```python
from build123d import *

# Parameters (mm, degrees)
BOSS_EXTRUDE1_DEPTH = 6
BOSS_EXTRUDE2_DEPTH = 1
BOSS_EXTRUDE3_START = 6
BOSS_EXTRUDE3_DEPTH = 6
SKETCH4_R           = 4
CUT_EXTRUDE1_DEPTH  = 0.7
SKETCH5_R           = 2
BOSS_EXTRUDE4_DEPTH = 0.7


with BuildPart() as part:
    # Sketch1 → Boss-Extrude1 (new body)
    with BuildSketch(Plane(origin=(0, 0, 0), x_dir=(1, 0, 0), z_dir=(0, 1, 0))):
        with BuildLine():
            ThreePointArc((-2.5, 7.282856582), (-7.7, 0), (-2.5, -7.282856582))
            Line((-2.5, -7.282856582), (-2.5, -6.216108107))
            ThreePointArc((-2.5, -6.216108107), (-6.7, 0), (-2.5, 6.216108107))
            Line((-2.5, 6.216108107), (-2.5, 7.282856582))
        make_face()
        with BuildLine():
            Line((-2.5, -6.216108107), (-2.5, -7.282856582))
            ThreePointArc((-2.5, -7.282856582), (0, -7.7), (2.5, -7.282856582))
            Line((2.5, -7.282856582), (2.5, -6.216108107))
            ThreePointArc((2.5, -6.216108107), (0, -6.7), (-2.5, -6.216108107))
        make_face()
        with BuildLine():
            Line((2.5, -6.216108107), (2.5, -7.282856582))
            ThreePointArc((2.5, -7.282856582), (6.266578014, -4.474371464), (7.7, 0))
            ThreePointArc((7.7, 0), (6.266578014, 4.474371464), (2.5, 7.282856582))
            Line((2.5, 7.282856582), (2.5, 6.216108107))
            ThreePointArc((2.5, 6.216108107), (5.551576353, 3.750999867), (6.7, 0))
            ThreePointArc((6.7, 0), (5.551576353, -3.750999867), (2.5, -6.216108107))
        make_face()
    extrude(amount=BOSS_EXTRUDE1_DEPTH)

    # Sketch2 → Boss-Extrude2 (add)
    with BuildSketch(Plane(origin=(0, 6, 0), x_dir=(1, 0, 0), z_dir=(0, 1, 0))):
        with BuildLine():
            Line((3, 13.7), (-3, 13.7))
            Line((-3, 13.7), (-7.191011254, 2.753063229))
            ThreePointArc((-7.191011254, 2.753063229), (-5.348708418, 5.539071968), (-2.5, 7.282856582))
            ThreePointArc((-2.5, 7.282856582), (0, 7.7), (2.5, 7.282856582))
            ThreePointArc((2.5, 7.282856582), (5.348708418, 5.539071968), (7.191011254, 2.753063229))
            Line((7.191011254, 2.753063229), (3, 13.7))
        make_face()
        with BuildLine():
            ThreePointArc((2.5, 6.216108107), (0, -6.7), (-2.5, 6.216108107))
            Line((-2.5, 6.216108107), (-2.5, 7.282856582))
            ThreePointArc((-2.5, 7.282856582), (0, -7.7), (2.5, 7.282856582))
            Line((2.5, 7.282856582), (2.5, 6.216108107))
        make_face()
        with BuildLine():
            ThreePointArc((-2.5, 7.282856582), (-5.348708418, 5.539071968), (-7.191011254, 2.753063229))
            ThreePointArc((-7.191011254, 2.753063229), (-1.399859519, -7.571683652), (7.7, 0))
            ThreePointArc((7.7, 0), (7.571683652, 1.399859519), (7.191011254, 2.753063229))
            ThreePointArc((7.191011254, 2.753063229), (5.348708418, 5.539071968), (2.5, 7.282856582))
            Line((2.5, 7.282856582), (2.5, 6.216108107))
            ThreePointArc((2.5, 6.216108107), (0, -6.7), (-2.5, 6.216108107))
            Line((-2.5, 6.216108107), (-2.5, 7.282856582))
        make_face()
        with BuildLine():
            ThreePointArc((2.5, 7.282856582), (0, 7.7), (-2.5, 7.282856582))
            Line((-2.5, 7.282856582), (-2.5, 6.216108107))
            ThreePointArc((-2.5, 6.216108107), (0, -6.7), (2.5, 6.216108107))
            Line((2.5, 6.216108107), (2.5, 7.282856582))
        make_face()
    extrude(amount=BOSS_EXTRUDE2_DEPTH)

    # Sketch3 → Boss-Extrude3 (add)
    with BuildSketch(Plane.XZ.offset(-6).offset(BOSS_EXTRUDE3_START)):
        with BuildLine():
            Line((-7.191011254, -2.753063229), (-3, -13.7))
            Line((-3, -13.7), (-1.929218753, -13.7))
            Line((-1.929218753, -13.7), (-2.5, -7.282856582))
            ThreePointArc((-2.5, -7.282856582), (-5.348708418, -5.539071968), (-7.191011254, -2.753063229))
        make_face()
        with BuildLine():
            Line((2.5, -7.282856582), (1.929218753, -13.7))
            Line((1.929218753, -13.7), (3, -13.7))
            Line((3, -13.7), (7.191011254, -2.753063229))
            ThreePointArc((7.191011254, -2.753063229), (5.348708418, -5.539071968), (2.5, -7.282856582))
        make_face()
    extrude(amount=-BOSS_EXTRUDE3_DEPTH)

    # Sketch4 → Cut-Extrude1 (cut)
    with BuildSketch(Plane(origin=(0, 7, 0), x_dir=(1, 0, 0), z_dir=(0, 1, 0))):
        Circle(SKETCH4_R)
        with BuildLine():
            Line((-2.031506006, 3.445719569), (-3.200269116, 4.473061322))
            ThreePointArc((-3.200269116, 4.473061322), (-3.889087297, 3.889087297), (-4.473061322, 3.200269116))
            Line((-4.473061322, 3.200269116), (-3.445719569, 2.031506006))
            ThreePointArc((-3.445719569, 2.031506006), (-2.828427125, 2.828427125), (-2.031506006, 3.445719569))
        make_face()
        with BuildLine():
            Line((-3.872983346, 1), (-5.425863987, 0.9))
            ThreePointArc((-5.425863987, 0.9), (-5.5, 0), (-5.425863987, -0.9))
            Line((-5.425863987, -0.9), (-3.872983346, -1))
            ThreePointArc((-3.872983346, -1), (-4, 0), (-3.872983346, 1))
        make_face()
        with BuildLine():
            Line((-3.445719569, -2.031506006), (-4.473061322, -3.200269116))
            ThreePointArc((-4.473061322, -3.200269116), (-3.889087297, -3.889087297), (-3.200269116, -4.473061322))
            Line((-3.200269116, -4.473061322), (-2.031506006, -3.445719569))
            ThreePointArc((-2.031506006, -3.445719569), (-2.828427125, -2.828427125), (-3.445719569, -2.031506006))
        make_face()
        with BuildLine():
            Line((-1, -3.872983346), (-0.9, -5.425863987))
            ThreePointArc((-0.9, -5.425863987), (0, -5.5), (0.9, -5.425863987))
            Line((0.9, -5.425863987), (1, -3.872983346))
            ThreePointArc((1, -3.872983346), (0, -4), (-1, -3.872983346))
        make_face()
        with BuildLine():
            ThreePointArc((3.200269116, -4.473061322), (3.889087297, -3.889087297), (4.473061322, -3.200269116))
            Line((4.473061322, -3.200269116), (3.445719569, -2.031506006))
            ThreePointArc((3.445719569, -2.031506006), (2.828427125, -2.828427125), (2.031506006, -3.445719569))
            Line((2.031506006, -3.445719569), (3.200269116, -4.473061322))
        make_face()
        with BuildLine():
            ThreePointArc((5.5, 0), (5.481434663, 0.451524127), (5.425863987, 0.9))
            Line((5.425863987, 0.9), (3.872983346, 1))
            ThreePointArc((3.872983346, 1), (3.968118785, 0.50401717), (4, 0))
            ThreePointArc((4, 0), (3.968118785, -0.50401717), (3.872983346, -1))
            Line((3.872983346, -1), (5.425863987, -0.9))
            ThreePointArc((5.425863987, -0.9), (5.481434663, -0.451524127), (5.5, 0))
        make_face()
        with BuildLine():
            ThreePointArc((4.473061322, 3.200269116), (3.889087297, 3.889087297), (3.200269116, 4.473061322))
            Line((3.200269116, 4.473061322), (2.031506006, 3.445719569))
            ThreePointArc((2.031506006, 3.445719569), (2.828427125, 2.828427125), (3.445719569, 2.031506006))
            Line((3.445719569, 2.031506006), (4.473061322, 3.200269116))
        make_face()
        with BuildLine():
            ThreePointArc((0.9, 5.425863987), (0, 5.5), (-0.9, 5.425863987))
            Line((-0.9, 5.425863987), (-1, 3.872983346))
            ThreePointArc((-1, 3.872983346), (0, 4), (1, 3.872983346))
            Line((1, 3.872983346), (0.9, 5.425863987))
        make_face()
    extrude(amount=-CUT_EXTRUDE1_DEPTH, mode=Mode.SUBTRACT)

    # Sketch5 → Boss-Extrude4 (add)
    with BuildSketch(Plane(origin=(0, 6.3, 0), x_dir=(1, 0, 0), z_dir=(0, 1, 0))):
        with Locations(Location((0, 0, 0), (0, 0, 270))):
            Circle(SKETCH5_R)
    extrude(amount=BOSS_EXTRUDE4_DEPTH)


solid = part.part
```
Could you check a few things on this model? Use its own coordinates, in mm. A direction names the side the tool comes from. Coordinates: 2 decimals unless noted, no trailing zeros. Loops run counter-clockwise (first coordinate to the right, second up) from the corner with the lowest first, then second, coordinate; pieces in that order, holes last.
1) Please list where these lines run through material, in increasing order: line 1 along X through (y, z) = (6.5, -1.25); line 2 along Y through (x, z) = (4.75, -4.25); line 3 along X through (y, z) = (3.5, -2).
Reported:
line 1: x = -7.6 to -3.8, -1.56 to 1.56, 3.8 to 7.6
line 2: y = 6 to 7
line 3: x = -7.44 to -6.39, 6.39 to 7.44
2) Imagine slicing it at B-B (x = 0). List the corners of the cut face in (y, z) for me, and give its area (3 significant figures).
Reported:
outline: (0, 6.7) - (6, 6.7) - (6, -13.7) - (7, -13.7) - (7, -5.5) - (6.3, -5.5) - (6.3, -2) - (7, -2) - (7, 2) - (6.3, 2) - (6.3, 5.5) - (7, 5.5) - (7, 7.7) - (0, 7.7) - close
area: 22.5 mm2
3) Imagine slicing it at D-D (x = -6.25). List the corners of the cut face in (y, z) for me.
Reported:
outline: (0, -5.21) - (7, -5.21) - (7, 4.5) - (0, 4.5) - (0, 2.41) - (6, 2.41) - (6, -2.41) - (0, -2.41) - close
4) Thinking about a two-plate mould opening in X: for faces 1 (the face through (0, 7, -6)), 2 (the face through (2.608, 6.655, 3.952)), 3 (the face through (2.4, 6.3, -0.1)), which applies, released by +X, released by -X, zero draft, split by the parting line, or undercut?
Reported:
face 1: zero draft
face 2: undercut
face 3: undercut
5) Imagine slicing it at C-C (z = -7.75). List the corners of the cut face in (x, y) for me, and give its area (3 significant figures).
Reported:
outline: (-5.28, 0) - (-2.46, 0) - (-2.46, 6) - (2.46, 6) - (2.46, 0) - (5.28, 0) - (5.28, 7) - (-5.28, 7) - close
area: 44.4 mm2
6) Imagine slicing it at A-A (y = 3.5). List the corners of the cut face in (x, z) for me.
Reported:
outline: (-7.19, -2.75) - (-3, -13.7) - (-1.93, -13.7) - (-2.5, -7.28) - (-2.5, -6.22) arc R6.7 cw (long way) to (2.5, -6.22) - (2.5, -7.28) - (1.93, -13.7) - (3, -13.7) - (7.19, -2.75) arc R7.7 ccw (long way) to start
7) Will these pins go through, and if not, where does the flat tip stop? pin 1 Ø0.9 at (y, z) = (1.5, -7) entering from +X; pin 2 Ø4 at (x, z) = (-3, -2) entering from -Y; pin 3 Ø4 at (y, z) = (1.5, -3) entering from +X.
Reported:
pin 1: stops at x = 5.74
pin 2: stops at y = 6
pin 3: stops at x = 7.63
8) Which directions (+Z, -Z, +X, -X, +Y, -Y) give clear straight access to the entire face, cutting with the end or side of a thin tool? Please do faces 4 (the face through (2.5, 3, -7)), 5 (the face through (3.88, 6.65, 3.9)).
Reported:
face 4: -Y
face 5: +Y
